Print and shaded views of the part. All mm, measured from the part's lowest x, y and z. A direction names the side the tool comes from. Coordinates: 2 decimals unless noted, no trailing zeros. Loops run counter-clockwise (first coordinate to the right, second up) from the corner with the lowest first, then second, coordinate; pieces in that order, holes last. Notation, with made-up numbers: M 21,-20.75 L 43,-20.75 A12 ccw 43,-9.75 Z; hole C -9,47.25 d7. An arc over 180 degrees is marked long. Use a Markdown table: item, result. Add a question column.
1) Tool access for the marked faces 1 and 2: list every direction of +Z, -Z, +X, -X, +Y, -Y with a clear straight run to the whole face (end or side of a thin tool).
2) Band-saw the part on B-B (x = 120). List the corners of the cut face in (y, z).
3) Pin check, flat tip, straight feed: pin 1 Ø4 at (x, y) = (100.5, 26) entering from +Z. Stop position of the tip, or through.
4) Band-saw the part on A-A (y = 46). List the corners of the cut face in (x, z).
5) Band-saw the part on C-C (z = 69). List the corners of the cut face in (x, y), plus the area to 3 significant figures.
6) Wall check: probe 1 along Z at (x, y) = (121.5, 84.5). Give the ranges that are in metal, low to high. Write a range as from..to.
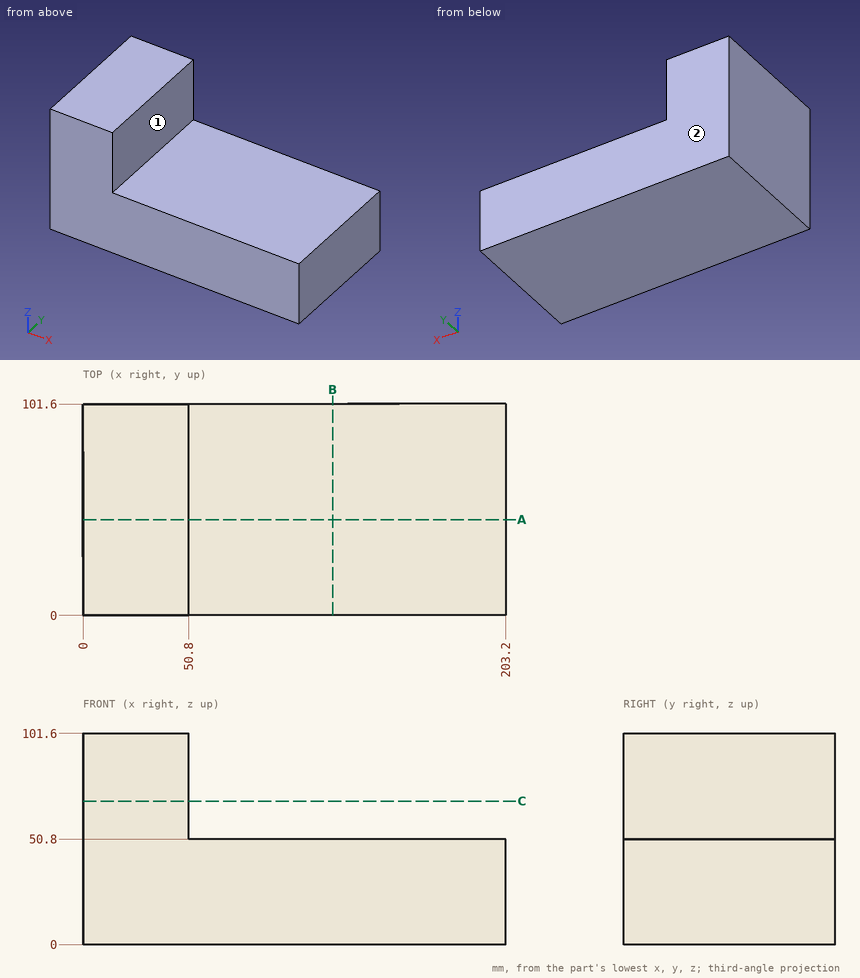
Entries:
| question | item | result |
|---|---|---|
| 1 | face 1 | +Z, +X, +Y, -Y |
| 1 | face 2 | +Z, -Z, +X, -X, +Y |
| 2 | outline | M 0,0 L 101.6,0 L 101.6,50.8 L 0,50.8 Z |
| 3 | pin 1 | z = 50.8 |
| 4 | outline | M 0,0 L 203.2,0 L 203.2,50.8 L 50.8,50.8 L 50.8,101.6 L 0,101.6 Z |
| 5 | outline | M 0,0 L 50.8,0 L 50.8,101.6 L 0,101.6 Z |
| 5 | area | 5,160 mm2 |
| 6 | probe 1 | 0..50.8 |
